For this review, use the dimensioned drawing (mm, ordinates from the lowest corner) and the shaded views. A direction names the side the tool comes from. Give positions to 0.01 mm unless a question says otherwise; leave off trailing zeros. Order: outer loops, then holes, each group sorted by start corner. A loop starts at its lowest first (then second) coordinate and runs counter-clockwise, first axis right, second up. Notation, with made-up numbers: M -3.75,-7.75 L 31.25,-7.75 A8 ccw 31.25,-1.75 Z; hole C 66,45.25 d10. An arc over 180 degrees is marked long. Use CSV: the item, a comma, the result in double quotes. Start each with the question number.
(1) Tool access review of the marked faces 1, 2 and 3: name each direction out of +Z, -Z, +X, -X, +Y, -Y from which nothing blocks a thin tool from reaching the whole face with its end or side.
(2) Wall thickness on L1, parallel to Y at x = 2.05, z = 10.5; L2, parallel to Z at x = 0.25, y = 13; L3, parallel to Y at x = 2.8, z = 2: over which ranges is each line inside the solid? List them lowest first. Write a range as from..to.
(3) Consider section D-D (y = 13.5). Write out the cut boundary in (x, z), and give its area (3 significant figures).
(4) Consider section C-C (x = 2.1). Write out the cut boundary in (y, z), and give its area (3 significant figures).
(5) Consider section A-A (y = 7.5). Write out the cut boundary in (x, z), and give its area (3 significant figures).
(6) Consider section B-B (z = 10.5). Write out the cut boundary in (x, y), and give its area (3 significant figures).
(7) Clearance check with flat-ended pins moving along their axes: P1, Ø1.2, axis at x = 1.5, y = 1, coming from the +Z side; P2, Ø0.9, axis at x = 2, z = 19, coming from the -Y side; P3, Ø0.9, axis at x = 2, z = 19, coming from the +Y side. State where each tip first meets the part, or that it passes through.
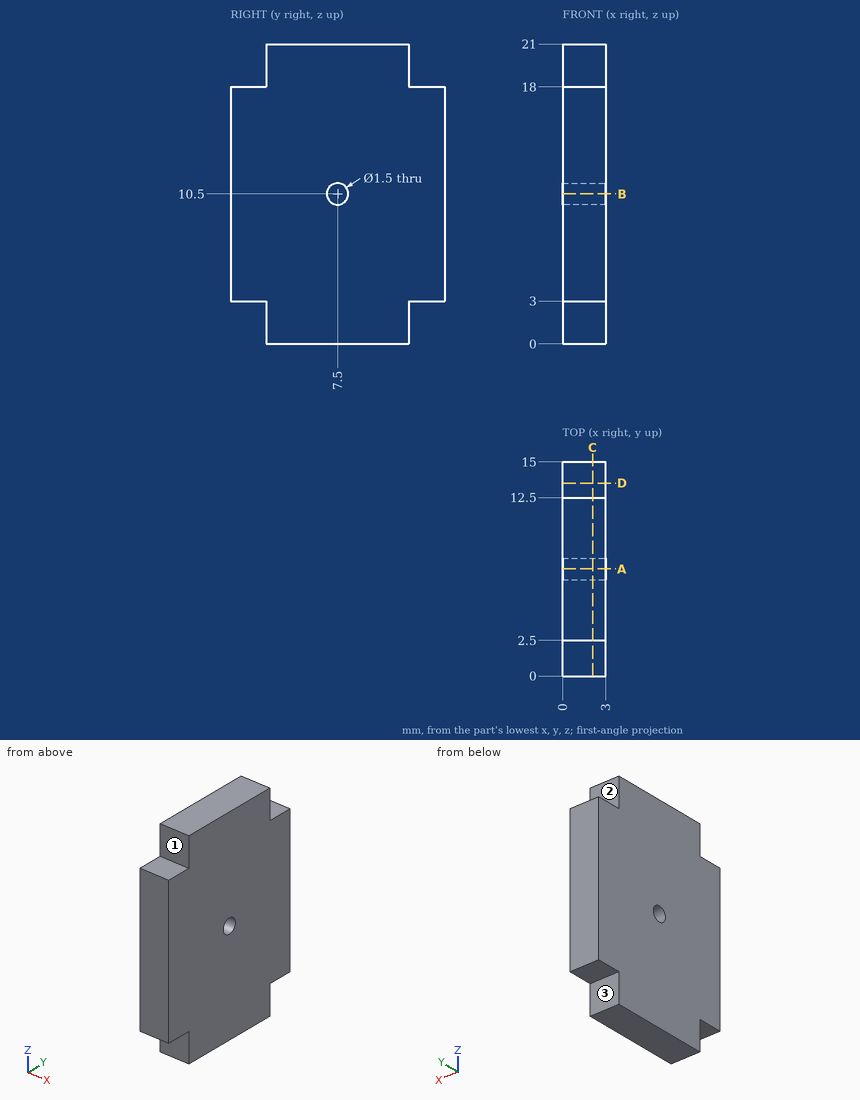
Check result:
1,face 1,"+Z, +X, -X, -Y"
1,face 2,"+Z, +X, -X, +Y"
1,face 3,"-Z, +X, -X, +Y"
2,L1,"y = 0..6.75, 8.25..15"
2,L2,"z = 3..18"
2,L3,"y = 2.5..12.5"
3,outline,"M 0,3 L 3,3 L 3,18 L 0,18 Z"
3,area,"45.0 mm^2"
4,outline,"M 0,3 L 2.5,3 L 2.5,0 L 12.5,0 L 12.5,3 L 15,3 L 15,18 L 12.5,18 L 12.5,21 L 2.5,21 L 2.5,18 L 0,18 Z; hole C 7.5,10.5 d1.5"
4,area,"283 mm^2"
5,outline,"M 0,0 L 3,0 L 3,9.75 L 0,9.75 Z; M 0,11.25 L 3,11.25 L 3,21 L 0,21 Z"
5,area,"58.5 mm^2"
6,outline,"M 0,0 L 3,0 L 3,6.75 L 0,6.75 Z; M 0,8.25 L 3,8.25 L 3,15 L 0,15 Z"
6,area,"40.5 mm^2"
7,P1,"stops at z = 18"
7,P2,"stops at y = 2.5"
7,P3,"stops at y = 12.5"
